```python
from build123d import *
from build123d.topology import SkipClean

# Parameters (mm, degrees)
SKETCH2_R               = 7.5
BOSS_EXTRUDE1_DEPTH     = 2.8
M3_CLEARANCE_HOLE1_D    = 3.2
M3X0_5_TAPPED_HOLE1_D   = 2.5
SKETCH8_R               = 1.25
SKETCH8_R_2             = 7.5
BOSS_EXTRUDE2_DEPTH     = 0.7
CUT_EXTRUDE1_DEPTH      = 46.416804125
CUT_EXTRUDE1_DEPTH_BACK = 46.416804125
FILLET3_R               = 2.5
MOVE_FACE2_BY           = 0.1
SKETCH18_R              = 1.25
SKETCH18_R_2            = 7.5
SKETCH18_R_3            = 1.6
BOSS_EXTRUDE5_DEPTH     = 3.4
MOVE_START              = -17
MOVE_FACE5_OUTLINE_W    = 42.925322608
MOVE_FACE5_OUTLINE_H    = 3.4
MOVE_FACE5_DEPTH        = 2
SKETCH19_R              = 4
CUT_EXTRUDE3_DEPTH      = 0.7
FILLET5_R               = 1
MOVE_FACE3_BY           = 0.2
MOVE_FACE4_BY           = 0.2
FILLET6_R               = 3
CUT_EXTRUDE4_DEPTH      = 47.958344273
SKETCH22_R              = 1.6
CUT_EXTRUDE7_DEPTH      = 47.958344273
SKETCH25_W              = 32
SKETCH25_H              = 15
BOSS_EXTRUDE6_DEPTH     = 3.2
M3_CLEARANCE_HOLE2_D    = 3.2
FILLET7_R               = 1


with BuildPart() as part:
    # Sketch2 → Boss-Extrude1 (new body)
    with BuildSketch(Plane.XY):
        with BuildLine():
            Line((27.745372612, -11.410271628), (3.991101213, 29.733333333))
            ThreePointArc((3.991101213, 29.733333333), (0, 34), (-3.991101213, 29.733333333))
            Line((-3.991101213, 29.733333333), (-27.745372612, -11.410271628))
            ThreePointArc((-27.745372612, -11.410271628), (-29.444863729, -17), (-23.7542714, -18.323061706))
            Line((-23.7542714, -18.323061706), (23.7542714, -18.323061706))
            ThreePointArc((23.7542714, -18.323061706), (29.444863729, -17), (27.745372612, -11.410271628))
        make_face()
        Circle(SKETCH2_R, mode=Mode.SUBTRACT)
    extrude(amount=BOSS_EXTRUDE1_DEPTH)

    # M3 Clearance Hole1 (through all)
    with Locations(Plane.XY.offset(2.8)):
        with Locations((0, 30), (-25.980762114, -15), (25.980762114, -15)):
            Hole(M3_CLEARANCE_HOLE1_D / 2)

    # M3x0.5 Tapped Hole1 (through all)
    with Locations(Plane(origin=(0, 0, 0), x_dir=(-1, 0, 0), z_dir=(0, 0, -1))):
        with Locations((10.392304845, -6), (0, 12), (-10.392304845, -6)):
            Hole(M3X0_5_TAPPED_HOLE1_D / 2)

    # Sketch8 → Boss-Extrude2 (add)
    with SkipClean():  # the faces are left unmerged after this step: merging them gives an invalid solid
        with BuildSketch(Plane(origin=(0, 0, 0), x_dir=(-1, 0, 0), z_dir=(0, 0, -1))):
            with BuildLine():
                Line((-3.464101615, 14), (-13.856406461, -4))
                ThreePointArc((-13.856406461, -4), (-13.856406461, -8), (-10.392304845, -10))
                Line((-10.392304845, -10), (10.392304845, -10))
                ThreePointArc((10.392304845, -10), (13.856406461, -8), (13.856406461, -4))
                Line((13.856406461, -4), (3.464101615, 14))
                ThreePointArc((3.464101615, 14), (0, 16), (-3.464101615, 14))
            make_face()
            with Locations((-10.392304845, -6)):
                Circle(SKETCH8_R, mode=Mode.SUBTRACT)
            with Locations((0, 12)):
                Circle(SKETCH8_R, mode=Mode.SUBTRACT)
            with Locations((10.392304845, -6)):
                Circle(SKETCH8_R, mode=Mode.SUBTRACT)
            Circle(SKETCH8_R_2, mode=Mode.SUBTRACT)
        extrude(amount=BOSS_EXTRUDE2_DEPTH)
    add(part.part.scale(1), mode=Mode.REPLACE)  # the faces are merged on a copy

    # Sketch9 → Cut-Extrude1 (cut, two sides: drawn at the far end of the back side and taken through both)
    with BuildSketch(Plane(origin=(0, 0, 0), x_dir=(-1, 0, 0), z_dir=(0, 0, -1)).offset(-CUT_EXTRUDE1_DEPTH_BACK)):
        Polygon((27.745372612, -11.410271628), (3.991101213, 29.733333333), (3.991101213, 17.087209922), (16.793508478, -5.087209922), align=None)
        Polygon((12.802407266, -12), (-12.802407266, -12), (-23.7542714, -18.323061706), (23.7542714, -18.323061706), align=None)
        Polygon((-16.793508478, -5.087209922), (-3.991101213, 17.087209922), (-3.991101213, 29.733333333), (-27.745372612, -11.410271628), align=None)
    extrude(amount=CUT_EXTRUDE1_DEPTH + CUT_EXTRUDE1_DEPTH_BACK, mode=Mode.SUBTRACT)

    # Fillet3
    fillet3_edges = [part.edges().sort_by_distance(p)[0] for p in [
        (3.991101213, 17.087209922, 1.4),
        (16.793508478, -5.087209922, 1.4),
        (12.802407266, -12, 1.4),
        (-12.802407266, -12, 1.4),
        (-16.793508478, -5.087209922, 1.4),
        (-3.991101213, 17.087209922, 1.4),
    ]]
    fillet(fillet3_edges, radius=FILLET3_R)

    # Move Face2: a face moved inward by 0.1
    extrude(part.faces().sort_by_distance((0, 20.75, 2.8))[0], amount=MOVE_FACE2_BY, dir=(0, 0, -1), mode=Mode.SUBTRACT)

    # Sketch18 → Boss-Extrude5 (add)
    with BuildSketch(Plane.XY.offset(2.7)):
        with BuildLine():
            Line((-17.998559688, -15), (17.998559688, -15))
            Line((17.998559688, -15), (23.7542714, -18.323061706))
            ThreePointArc((23.7542714, -18.323061706), (29.444863729, -17), (27.745372612, -11.410271628))
            Line((27.745372612, -11.410271628), (21.989660901, -8.087209922))
            Line((21.989660901, -8.087209922), (16, 2.287187079))
            Line((16, 2.287187079), (16, 36))
            Line((16, 36), (-16, 36))
            Line((-16, 36), (-16, 2.287187079))
            Line((-16, 2.287187079), (-21.989660901, -8.087209922))
            Line((-21.989660901, -8.087209922), (-27.745372612, -11.410271628))
            ThreePointArc((-27.745372612, -11.410271628), (-29.444863729, -17), (-23.7542714, -18.323061706))
            Line((-23.7542714, -18.323061706), (-17.998559688, -15))
        make_face()
        with Locations(Location((0, 12, 0), (0, 0, 180))):
            Circle(SKETCH18_R, mode=Mode.SUBTRACT)
        with Locations(Location((10.392304845, -6, 0), (0, 0, 180))):
            Circle(SKETCH18_R, mode=Mode.SUBTRACT)
        with Locations(Location((-10.392304845, -6, 0), (0, 0, 180))):
            Circle(SKETCH18_R, mode=Mode.SUBTRACT)
        with Locations(Location((0, 0, 0), (0, 0, 180))):
            Circle(SKETCH18_R_2, mode=Mode.SUBTRACT)
        with Locations((0, 30)):
            Circle(SKETCH18_R_3, mode=Mode.SUBTRACT)
        with Locations((-25.980762114, -15)):
            Circle(SKETCH18_R_3, mode=Mode.SUBTRACT)
        with Locations((25.980762114, -15)):
            Circle(SKETCH18_R_3, mode=Mode.SUBTRACT)
    extrude(amount=-BOSS_EXTRUDE5_DEPTH)

    # Move Face5: read off the stored shape, not the designer's step
    # Move Face5 outline → Move Face5 (add)
    with BuildSketch(Plane(origin=(0, 0, 0), x_dir=(1, 0, 0), z_dir=(0, 1, 0)).offset(MOVE_START)):
        with Locations((0, -1)):
            Rectangle(MOVE_FACE5_OUTLINE_W, MOVE_FACE5_OUTLINE_H)
    extrude(amount=MOVE_FACE5_DEPTH)

    # Sketch19 → Cut-Extrude3 (cut)
    with BuildSketch(Plane(origin=(0, 0, -0.7), x_dir=(-1, 0, 0), z_dir=(0, 0, -1))):
        with Locations((25.980762114, -15)):
            Circle(SKETCH19_R)
        with Locations((-25.980762114, -15)):
            Circle(SKETCH19_R)
        with Locations((0, 30)):
            Circle(SKETCH19_R)
    extrude(amount=-CUT_EXTRUDE3_DEPTH, mode=Mode.SUBTRACT)

    # Fillet5
    # the kernel refuses this fillet: 1 mm, written as the material it takes off along each edge
    with BuildSketch(Plane(origin=(-23.7542714, -18.323061706, 0), x_dir=(0.5630065866190214, 0.8264524084444297, 0), z_dir=(0, 0, -1)), Plane(origin=(23.7542714, -18.323061706, -8.164117066), x_dir=(-0.5630065866190195, 0.826452408444431, -1.7271463390342054e-15), z_dir=(0, 0, 1))) as fillet5_piece_1:
        with BuildLine():
            CenterArc((3.35885268, 0.92774856), FILLET5_R, 167.216617388, 80.869915665)
            Line((2.383639111, 1.149014228), (0, 0))
            ThreePointArc((0, 0), (1.492823413, 0.289005759), (2.985646826, 0))
        make_face()
    extrude(amount=8.164117066, mode=Mode.SUBTRACT)
    with BuildSketch(Plane(origin=(-27.745372612, -11.410271628, 0), x_dir=(0.9996753598266718, 0.025478911974695106, 0), z_dir=(0, 0, -1)), Plane(origin=(27.745372612, -11.410271628, -10.049979958), x_dir=(-0.9996753598266713, 0.02547891197471748, -2.7505093848186077e-14), z_dir=(0, 0, 1))) as fillet5_piece_2:
        with BuildLine():
            CenterArc((3.763294339, -0.90838084), FILLET5_R, 114.717454154, 126.742537963)
            Line((3.285522044, -1.786864553), (0, 0))
            ThreePointArc((0, 0), (1.672575262, -0.366476642), (3.345150524, 0))
        make_face()
    extrude(amount=10.049979958, mode=Mode.SUBTRACT)
    with BuildSketch(Plane(origin=(-16, 36, 5.2), x_dir=(0, -1, 0), z_dir=(0, 0, -1)), Plane(origin=(16, 36, 5.2), x_dir=(-1, 0, 0), z_dir=(0, 0, -1))) as fillet5_piece_3:
        with BuildLine():
            CenterArc((FILLET5_R, -FILLET5_R), FILLET5_R, 90, 90)
            Line((0, -FILLET5_R), (0, 0))
            Line((0, 0), (FILLET5_R, 0))
        make_face()
    extrude(amount=8.4, mode=Mode.SUBTRACT)

    # Move Face3: a curved face moved inward by 0.2
    add(Solid.thicken(part.faces().sort_by_distance((4, 30, -0.35))[0], -MOVE_FACE3_BY), mode=Mode.SUBTRACT)

    # Move Face4: a face moved inward by 0.2
    extrude(part.faces().sort_by_distance((0, 8.5, 2.7))[0], amount=MOVE_FACE4_BY, dir=(0, 0, -1), mode=Mode.SUBTRACT)

    # Fillet6
    fillet6_edges = [part.edges().sort_by_distance(p)[0] for p in [
        (-21.989660901, -8.087209922, 0.9),
        (21.989660901, -8.087209922, 0.9),
        (21.462661304, -17, 1.25),
        (16, 2.287187079, 0.9),
        (-16, 2.287187079, 0.9),
        (-21.462661304, -17, 1.25),
    ]]
    fillet(fillet6_edges, radius=FILLET6_R)

    # Sketch20 → Cut-Extrude4 (cut, through all)
    with BuildSketch(Plane(origin=(0, 0, -0.7), x_dir=(-1, 0, 0), z_dir=(0, 0, -1))):
        with BuildLine():
            Line((14.6, 33), (14.6, 29))
            ThreePointArc((14.6, 29), (13, 27.4), (11.4, 29))
            Line((11.4, 29), (11.4, 33))
            ThreePointArc((11.4, 33), (13, 34.6), (14.6, 33))
        make_face()
        with BuildLine():
            Line((11.4, 21), (11.4, 17))
            ThreePointArc((11.4, 17), (13, 15.4), (14.6, 17))
            Line((14.6, 17), (14.6, 21))
            ThreePointArc((14.6, 21), (13, 22.6), (11.4, 21))
        make_face()
        with BuildLine():
            Line((11.4, 9), (11.4, 5))
            ThreePointArc((11.4, 5), (13, 3.4), (14.6, 5))
            Line((14.6, 5), (14.6, 9))
            ThreePointArc((14.6, 9), (13, 10.6), (11.4, 9))
        make_face()
        with BuildLine():
            Line((-14.6, 33), (-14.6, 29))
            ThreePointArc((-14.6, 29), (-13, 27.4), (-11.4, 29))
            Line((-11.4, 29), (-11.4, 33))
            ThreePointArc((-11.4, 33), (-13, 34.6), (-14.6, 33))
        make_face()
        with BuildLine():
            Line((-14.6, 21), (-14.6, 17))
            ThreePointArc((-14.6, 17), (-13, 15.4), (-11.4, 17))
            Line((-11.4, 17), (-11.4, 21))
            ThreePointArc((-11.4, 21), (-13, 22.6), (-14.6, 21))
        make_face()
        with BuildLine():
            Line((-14.6, 9), (-14.6, 5))
            ThreePointArc((-14.6, 5), (-13, 3.4), (-11.4, 5))
            Line((-11.4, 5), (-11.4, 9))
            ThreePointArc((-11.4, 9), (-13, 10.6), (-14.6, 9))
        make_face()
    extrude(amount=-CUT_EXTRUDE4_DEPTH, mode=Mode.SUBTRACT)

    # Sketch22 → Cut-Extrude7 (cut, through all)
    with BuildSketch(Plane(origin=(0, 0, -0.7), x_dir=(-1, 0, 0), z_dir=(0, 0, -1))):
        with Locations((13, -14)):
            Circle(SKETCH22_R)
        with Locations((-13, -14)):
            Circle(SKETCH22_R)
    extrude(amount=-CUT_EXTRUDE7_DEPTH, mode=Mode.SUBTRACT)

    # Sketch25 → Boss-Extrude6 (add)
    with BuildSketch(Plane(origin=(0, 0, -0.7), x_dir=(-1, 0, 0), z_dir=(0, 0, -1))):
        with Locations((0, -24.5)):
            Rectangle(SKETCH25_W, SKETCH25_H)
    extrude(amount=-BOSS_EXTRUDE6_DEPTH)

    # M3 Clearance Hole2 (through all)
    with Locations(Plane(origin=(0, 0, -0.7), x_dir=(-1, 0, 0), z_dir=(0, 0, -1))):
        with Locations((-13, -29), (13, -29)):
            Hole(M3_CLEARANCE_HOLE2_D / 2)

    # Fillet7
    fillet7_edges = [part.edges().sort_by_distance(p)[0] for p in [
        (-16, -32, 0.9),
        (-16, -17, 0.9),
        (16, -17, 0.9),
        (16, -32, 0.9),
    ]]
    fillet(fillet7_edges, radius=FILLET7_R)


solid = part.part
```
The listing builds one solid part. Answer for the finished solid, in the listing's coordinates (mm). A direction names the side the tool comes from. Coordinates: 2 decimals unless noted, no trailing zeros. Write each loop counter-clockwise with the first axis right and the second up, starting at its lowest first coordinate (ties: lowest second). Pieces come first, ordered by that corner, then holes. Notation, with made-up numbers: (36, 36.25) - (80, 36.25) arc R12 ccw to (80, 44.25) - close; hole circle Ø2 at (73.25, 60.25). An arc over 180 degrees is marked (long way). Return JSON: item names as keys, results as strings. Group by question number.
1. Given pin 1 (1 mm diameter, centred on y = 21.5, z = -0.5, fed in from -X); pin 2 (3 mm diameter, centred on x = 10.39, y = -6, fed in from +Z); pin 3 (1 mm diameter, centred on y = -26, z = 0.5, fed in from +X); pin 4 (0.6 mm diameter, centred on x = 25.5, y = -10.5, fed in from -Z), each flat-ended and moving along its own axis, determine where each tip first touches the part or whether it passes through.
2. Determine the mould class of faces 1 (the cylindrical face through (-11.4, -13.93, 0.88)), 2 (the flat face through (19.03, -2.96, 0.92)), 3 (the flat face through (5, -6, -0.7)) for opening direction X: released by +X, released by -X, zero draft, split by the parting line, or undercut.
3. A cutting plane is placed at A-A, the plane y = -29. Determine the outline of the cut face in (x, z), plus the area to 3 significant figures.
4. Straight lines are drawn through the part: L1, parallel to X at y = 19.5, z = -0.1; L2, parallel to Y at x = 12.5, z = 1.5; L3, parallel to X at y = -6, z = -0.25. For each, find the intervals that lie inside material, in ascending order.
5. A cutting plane is placed at C-C, the plane z = 1.25. Give the number of separate pieces and of enclosed holes in the cut face, plus the area to 3 significant figures.
6. Which of the six approach directions +Z, -Z, +X, -X, +Y, -Y give full straight-line access (tool end or side, diameter ignored) to faces 4 (the flat face through (-14.6, 31, 1)), 5 (the flat face through (16, 19, 1)), 6 (the flat face through (-22.97, -17.87, 1.27))?
7. A cutting plane is placed at B-B, the plane x = 13. Determine the outline of the cut face in (y, z), plus the area to 3 significant figures.
Ans:
{
 "1": {"pin 1": "x = -16", "pin 2": "z = 2.5", "pin 3": "x = 16", "pin 4": "z = 0"},
 "2": {"face 1": "undercut", "face 2": "released by +X", "face 3": "zero draft"},
 "3": {"outline": "(-16, -0.7) - (-14.6, -0.7) - (-14.6, 2.5) - (-16, 2.5) - close; (-11.4, -0.7) - (11.4, -0.7) - (11.4, 2.5) - (-11.4, 2.5) - close; (14.6, -0.7) - (16, -0.7) - (16, 2.5) - (14.6, 2.5) - close", "area": "81.9 mm²"},
 "4": {"L1": "-16 to -14.6, -11.4 to 11.4, 14.6 to 16", "L2": "-32 to -30.52, -27.48 to -15.52, -12.48 to 3.48, 10.52 to 15.48, 22.52 to 27.48, 34.52 to 36", "L3": "-20.78 to -11.64, -9.14 to -4.5, 4.5 to 9.14, 11.64 to 20.78"},
 "5": {"separate pieces": "1", "enclosed holes": "17", "area": "2,100 mm²"},
 "6": {"face 4": "+Z, -Z", "face 5": "+Z, -Z, +X, +Y", "face 6": "+Z, -Z, -Y"},
 "7": {"outline": "(-32, -0.7) - (-30.6, -0.7) - (-30.6, 2.5) - (-32, 2.5) - close; (-27.4, -0.7) - (-15.6, -0.7) - (-15.6, 2.5) - (-27.4, 2.5) - close; (-12.4, -0.7) - (3.4, -0.7) - (3.4, 2.5) - (-12.4, 2.5) - close; (10.6, -0.7) - (15.4, -0.7) - (15.4, 2.5) - (10.6, 2.5) - close; (22.6, -0.7) - (27.4, -0.7) - (27.4, 2.5) - (22.6, 2.5) - close; (34.6, -0.7) - (36, -0.7) - (36, 2.5) - (34.6, 2.5) - close", "area": "128 mm²"}
}
